from build123d import *

# Parameters (mm, degrees)
CROQUIS1_R              = 14.345
SALIENTE_EXTRUIR1_DEPTH = 3.5
CROQUIS2_R              = 36.845
SALIENTE_EXTRUIR2_DEPTH = 3


with BuildPart() as part:
    # Croquis1 → Saliente-Extruir1 (new body)
    with BuildSketch(Plane(origin=(0, 0, 0), x_dir=(0, 0, -1), z_dir=(1, 0, 0))):
        Circle(CROQUIS1_R)
        Polygon((7.332348419, 0), (3.666174209, 6.35), (-3.666174209, 6.35), (-7.332348419, 0), (-3.666174209, -6.35), (3.666174209, -6.35), align=None, mode=Mode.SUBTRACT)
    extrude(amount=SALIENTE_EXTRUIR1_DEPTH)

    # Croquis2 → Saliente-Extruir2 (add)
    with BuildSketch(Plane(origin=(3.5, 0, 0), x_dir=(0, 0, -1), z_dir=(1, 0, 0))):
        Circle(CROQUIS2_R)
        Polygon((7.332348419, 0), (3.666174209, 6.35), (-3.666174209, 6.35), (-7.332348419, 0), (-3.666174209, -6.35), (3.666174209, -6.35), align=None, mode=Mode.SUBTRACT)
    extrude(amount=SALIENTE_EXTRUIR2_DEPTH)


solid = part.part
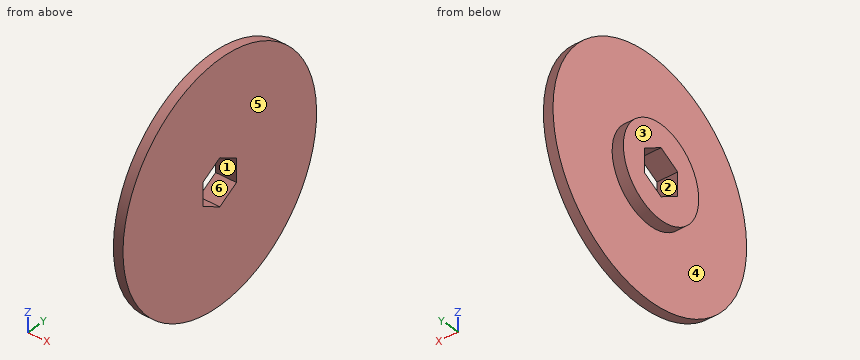
Build history of the part. All positions in model axes, mm. Face numbers are marked on the shaded views. A direction names the side the tool comes from. Coordinates: 2 decimals unless noted, no trailing zeros. Order: outer loops, then holes, each group sorted by start corner. A loop starts at its lowest first (then second) coordinate and runs counter-clockwise, first axis right, second up. Notation, with made-up numbers: (61, 29) - (80, 29) arc R10 ccw to (80, 42) - close; hole circle Ø10 at (14.5, 27.5). An arc over 180 degrees is marked (long way). Write each question's results on one line, items separated by ' | '. Start each with the question number.
Item 1: Band-saw the part on C-C on y = -9. Write the cut outline in (x, z).
Item 2: Mould opens along Y. For the marked faces 1, 2 and 3 say: released by +Y, released by -Y, zero draft, split by the parting line, or undercut.
Item 3: Band-saw the part on B-B on x = 5.25. Write the cut outline in (y, z) (3 decimals), and give its area (3 significant figures).
Item 4: Band-saw the part on A-A on z = 0. Write the cut outline in (x, y) (3 decimals).
Item 5: Band-saw the part on D-D on z = -27.5. Write the cut outline in (x, y).
Item 6: Tool access for the marked faces 4, 5 and 6: list every direction of +Z, -Z, +X, -X, +Y, -Y with a clear straight run to the whole face (end or side of a thin tool).
Item 7: Flat gauge pins, fed straight in: pin 1 (3 mm diameter, centred on x = 5.5, y = 23, fed in from +Z); pin 2 (22 mm diameter, centred on y = 17.5, z = 5, fed in from -X); pin 3 (3 mm diameter, centred on x = 1.5, z = 7.5, fed in from +Y). Where does each tip first touch, or does it go through?
Item 8: Wall check: probe 1 along Y at (x, z) = (5.25, -1); probe 2 along X at (y, z) = (-0.5, 32); probe 3 along Y at (x, z) = (0.5, -5.5). Give the ranges that are in metal, low to high. Write a range as [from, to].
Numbers:
1) outline: (0, -11.17) - (3.5, -11.17) - (3.5, -35.73) - (6.5, -35.73) - (6.5, 35.73) - (3.5, 35.73) - (3.5, 11.17) - (0, 11.17) - close
2) face 1: undercut | face 2: undercut | face 3: zero draft
3) outline: circle Ø73.69 at (0, 0); hole (-6.35, -3.666) - (0, -7.332) - (6.35, -3.666) - (6.35, 3.666) - (0, 7.332) - (-6.35, 3.666) - close | area: 4,130 mm^2
4) outline: (0, -14.345) - (3.5, -14.345) - (3.5, -36.845) - (6.5, -36.845) - (6.5, -6.35) - (0, -6.35) - close; (0, 6.35) - (6.5, 6.35) - (6.5, 36.845) - (3.5, 36.845) - (3.5, 14.345) - (0, 14.345) - close
5) outline: (3.5, -24.52) - (6.5, -24.52) - (6.5, 24.52) - (3.5, 24.52) - close
6) face 4: -X | face 5: +Z, -Z, +X, +Y, -Y | face 6: +X, -X
7) pin 1: z = 29.92 | pin 2: x = 0 | pin 3: y = 13.03
8) probe 1: [-36.83, -6.35], [6.35, 36.83] | probe 2: [3.5, 6.5] | probe 3: [-13.25, -3.17], [3.17, 13.25]
